Source: CAD feature listing. Evaluate the final solid. Frame: model axes, mm. Face numbers are marked on the shaded views. A direction names the side the tool comes from. Coordinates: 2 decimals unless noted, no trailing zeros. Loops run counter-clockwise (first coordinate to the right, second up) from the corner with the lowest first, then second, coordinate; pieces in that order, holes last.
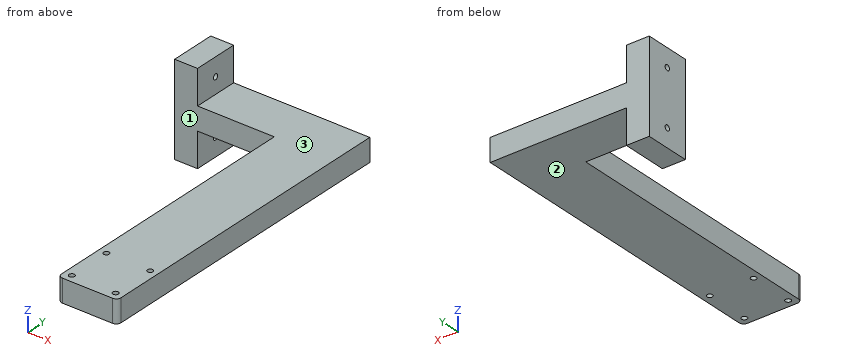
Autodesk Inventor part; units mm, degrees
ref_plane "YZ Plane" through (0, 0, 0) normal (1, 0, 0) x (0, 1, 0)
ref_plane "XZ Plane" through (0, 0, 0) normal (0, 1, 0) x (-1, 0, 0)
ref_plane "XY Plane" through (0, 0, 0) normal (0, 0, 1) x (1, 0, 0)
sketch "Sketch1" plane through (0, 0, 0) normal (0, 0, 1) x (1, 0, 0)
  line L0 (11.35, 40) -> (11.35, -15)
  line L1 (6.35, -20) -> (-48.65, -20)
  circle A0 centre (2.814466, -11.464466) radius 3
  circle A1 centre (-45.114466, -11.464466) radius 3
  circle A2 centre (-45.114466, 36.464466) radius 3
  circle A3 centre (2.814466, 36.464466) radius 3
  line L2 (-162.568945, -644.9995) -> (-162.568945, 135.0005)
  line L3 (11.35, -15) -> (11.35, 330)
  line L4 (-53.65, -15) -> (-53.65, 40)
  line L5 (-53.65, -15) -> (-53.65, 280)
  line L6 (11.35, 330) -> (-162.568945, 330)
  line L7 (-162.568945, 330) -> (-162.568945, 280)
  line L8 (-162.568945, 280) -> (-53.65, 280)
  line L9 (6.35, -20) -> (-48.65, -20)
  arc A4 (6.35, -20) -> (11.35, -15) centre (6.35, -15) ccw
  arc A5 (-53.65, -15) -> (-48.65, -20) centre (-48.65, -15) ccw
  circle A6 centre (2.814466, 36.464466) radius 3
  circle A7 centre (2.814466, -11.464466) radius 3
  circle A8 centre (-45.114466, -11.464466) radius 3
  circle A9 centre (-45.114466, 36.464466) radius 3
  point P0 (0, 0)
  dimension "d0" = 350
  dimension "d1" = 300
  dimension "d2" = 5
sketch "Sketch2" plane through (-162.568945, 280, 0) normal (-1, 0, 0) x (0, 0, 1)
  line L0 (0, 0) -> (25, 0)
  line L1 (0, 50) -> (25, 50)
  line L2 (25, 0) -> (25, 50)
  line L3 (-37.5, 50) -> (62.5, 50)
  line L4 (62.5, 50) -> (62.5, 0)
  line L5 (62.5, 0) -> (-37.5, 0)
  line L6 (-37.5, 0) -> (-37.5, 50)
  circle A0 centre (42.5, 25) radius 3
  circle A1 centre (-17.5, 25) radius 3
  point P0 (0, -280)
  point P1 (12.5, 50)
  point P2 (12.5, 50)
  point P3 (62.5, 25)
  point P4 (-37.5, 25)
  dimension "d4" = 50
  dimension "d5" = 50
  dimension "d6" = 25
  dimension "d7" = 20
  dimension "d8" = 20
  dimension "d9" = 6
sketch "Sketch1 outline for Plate1" plane through (0, 0, 0) normal (0, 0, 1) x (1, 0, 0)
  arc A0 (6.35, -20) -> (11.35, -15) centre (6.35, -15) ccw
  line L0 (-48.65, -20) -> (6.35, -20)
  line L1 (11.35, -15) -> (11.35, 330)
  arc A1 (-53.65, -15) -> (-48.65, -20) centre (-48.65, -15) ccw
  line L2 (11.35, 330) -> (-162.568945, 330)
  line L3 (-53.65, 280) -> (-53.65, -15)
  line L4 (-162.568945, 330) -> (-162.568945, 280)
  line L5 (-162.568945, 280) -> (-53.65, 280)
  circle A2 centre (-45.114466, -11.464466) radius 3
  circle A3 centre (2.814466, -11.464466) radius 3
  circle A4 centre (-45.114466, 36.464466) radius 3
  circle A5 centre (2.814466, 36.464466) radius 3
extrude "Plate1" add sketch "Sketch1 outline for Plate1" along normal blind 25
sketch "Sketch2 outline for Plate2" plane through (-162.568945, 280, 0) normal (-1, 0, 0) x (0, 0, 1)
  line L0 (-37.5, 50) -> (62.5, 50)
  line L1 (-37.5, 0) -> (-37.5, 50)
  line L2 (62.5, 50) -> (62.5, 0)
  line L3 (62.5, 0) -> (-37.5, 0)
  circle A0 centre (-17.5, 25) radius 3
  circle A1 centre (42.5, 25) radius 3
sheet face with bend "Face2" sketch "Sketch2 outline for Plate2" thickness 25 toward (1, 0, 0) bend radius 25
bend "Bend1"
equation "\"d3\" = Thickness"
equation "\"d10\" = BendRadius"
equation "\"d11\" = BendReliefWidth"
equation "\"d13\" = MinimumRemnant"
equation "\"d12\" = BendReliefDepth"
equation "\"d14\" = TransitionRadius"
equation "\"BendRadius\" = Thickness"
equation "\"BendReliefWidth\" = Thickness"
equation "\"BendReliefDepth\" = 0.5 * Thickness"
equation "\"TransitionRadius\" = BendRadius"
equation "\"JacobiRadiusSize\" = BendRadius"
equation "\"GapSize\" = Thickness"
properties part number "patas2"
Q1. Section query A-A on y = 112. Return the cut outline in (x, z), then the cut area to 4 significant figures.
Q2. Material intervals for line 1 along Z through (x, y) = (-151.25, 305); line 2 along Y through (x, z) = (-44.5, 15.5); line 3 along Y through (x, z) = (-154, -17), sorted ascending.
Q3. Section query B-B on x = -104.5. Return the cut outline in (y, z), then the cut area to 3 significant figures.
Q4. Reachability of the marked faces 1, 2 and 3 from +Z, -Z, +X, -X, +Y, -Y: full face, straight path, thin tool, end or side. Return the list, or none.
Q5. First-contact query: pin 1 Ø2 at (x, z) = (-88.5, 18.5) entering from -Y; pin 2 Ø12.5 at (y, z) = (108, 8) entering from -X; pin 3 Ø19 at (y, z) = (293, 38.5) entering from +X. Flat tips, straight axial feed; report the tip coordinate or a pass-through.
Resolved:
1. outline: (-53.65, 0) - (11.35, 0) - (11.35, 25) - (-53.65, 25) - close
1. area: 1,625 mm2
2. line 1: z = -37.5 to -20.5, -14.5 to 39.5, 45.5 to 62.5
2. line 2: y = -20 to -14.4, -8.53 to 33.53, 39.4 to 330
2. line 3: y = 280 to 302.04, 307.96 to 330
3. outline: (280, 0) - (330, 0) - (330, 25) - (280, 25) - close
3. area: 1,250 mm2
4. face 1: +Z, -Z, -X, -Y
4. face 2: -Z, +X, +Y, -Y
4. face 3: +Z, +X, +Y, -Y
5. pin 1: stops at y = 280
5. pin 2: stops at x = -53.65
5. pin 3: stops at x = -137.57
